Work out the finished part from the listing and answer in its coordinate system (mm). Face numbers are marked on the shaded views. A direction names the side the tool comes from. Round coordinates to 2 decimals unless told otherwise and drop trailing zeros. Loops run counter-clockwise (first coordinate to the right, second up) from the corner with the lowest first, then second, coordinate; pieces in that order, holes last. Notation, with made-up numbers: (-3, 33.25) - (10, 33.25) arc R16 cw to (10, 53.25) - close; hole circle Ø7 at (60, 45). An arc over 180 degrees is marked (long way). Answer as CSV lines item,"result". Start each with the question number.
Q1. For the marked faces 1 and 2, determine the directions among +Z, -Z, +X, -X, +Y, -Y from which every point of the face is accessible in a straight line to the end or side of a thin tool.
Q2. Section A-A on y = 0 is taken. Write down the section's boundary in (x, z).
Q3. Straight lines are drawn through the part: L1, parallel to Z at x = 14, y = 10.5; L2, parallel to Y at x = 0, z = 11; L3, parallel to Y at x = 0, z = 8. For each, find the intervals that lie inside material, in ascending order. Write a range as [from, to].
Q4. Each of these flat-tipped pins is pushed along its axis until it touches: pin 1 Ø3 at (x, z) = (1, 4) entering from -Y; pin 2 Ø4 at (y, z) = (-9.5, 8.5) entering from -X; pin 3 Ø1.5 at (x, y) = (-12, -11) entering from -Z. Where does it stop, or does it pass through?
Q5. Section C-C on z = 6 is taken. Write down the section's boundary in (x, y).
Q6. Section D-D on z = -8 is taken. Write down the section's boundary in (x, y), then the cut area to 3 significant figures.
Q7. Section B-B on x = 10 is taken. Write down the section's boundary in (y, z).
Q8. The mould has two halves that part along X. Classify the marked faces 3, 4 and 5: +X half, -X half, draft (parallel to the pull), parting line (faces both ways), or undercut.
```python
from build123d import *

# Parameters (mm, degrees)
SKETCH_1_R          = 18.5
SKETCH_1_R_2        = 3
EXTRUDE_1_DEPTH     = 14
SKETCH_2_R          = 18.5
SKETCH_2_R_2        = 17.3
CUT_EXTRUDE_1_DEPTH = 2.2
SKETCH_2_2_R        = 18.5
SKETCH_2_2_R_2      = 17.3
CUT_EXTRUDE_2_DEPTH = 0.8
SKETCH_2_4_R        = 18.5
SKETCH_2_4_R_2      = 17.3
CUT_EXTRUDE_3_DEPTH = 4
SKETCH_2_6_R        = 18.5
SKETCH_2_6_R_2      = 17.3
CUT_EXTRUDE_5_DEPTH = 3
SKETCH_3_R          = 7
EXTRUDE_3_DEPTH     = 5
SKETCH_4_R          = 6
EXTRUDE_4_DEPTH     = 12


with BuildPart() as part:
    # Sketch 1 → Extrude 1 (new body)
    with BuildSketch(Plane.XY):
        Circle(SKETCH_1_R)
        Circle(SKETCH_1_R_2, mode=Mode.SUBTRACT)
    extrude(amount=EXTRUDE_1_DEPTH)

    # Sketch 2 → Cut-Extrude 1 (cut)
    with BuildSketch(Plane.XY.offset(7.7)):
        Circle(SKETCH_2_R)
        Circle(SKETCH_2_R_2, mode=Mode.SUBTRACT)
    extrude(amount=-CUT_EXTRUDE_1_DEPTH, mode=Mode.SUBTRACT)

    # Sketch 2_2 → Cut-Extrude 2 (cut)
    with BuildSketch(Plane.XY.offset(7.7)):
        Circle(SKETCH_2_2_R)
        Circle(SKETCH_2_2_R_2, mode=Mode.SUBTRACT)
    extrude(amount=CUT_EXTRUDE_2_DEPTH, mode=Mode.SUBTRACT)

    # Sketch 2_4 → Cut-Extrude 3 (cut)
    with BuildSketch(Plane.XY.offset(7.7)):
        Circle(SKETCH_2_4_R)
        Circle(SKETCH_2_4_R_2, mode=Mode.SUBTRACT)
    extrude(amount=-CUT_EXTRUDE_3_DEPTH, mode=Mode.SUBTRACT)

    # Sketch 2_6 → Cut-Extrude 5 (cut)
    with BuildSketch(Plane.XY.offset(7.7)):
        Circle(SKETCH_2_6_R)
        Circle(SKETCH_2_6_R_2, mode=Mode.SUBTRACT)
    extrude(amount=CUT_EXTRUDE_5_DEPTH, mode=Mode.SUBTRACT)

    # Sketch 3 → Extrude 3 (add)
    with BuildSketch(Plane(origin=(0, 0, 0), x_dir=(-1, 0, 0), z_dir=(0, 0, -1))):
        Circle(SKETCH_3_R)
    extrude(amount=EXTRUDE_3_DEPTH)

    # Sketch 4 → Extrude 4 (add)
    with BuildSketch(Plane(origin=(0, 0, -5), x_dir=(-1, 0, 0), z_dir=(0, 0, -1))):
        Circle(SKETCH_4_R)
    extrude(amount=EXTRUDE_4_DEPTH)


solid = part.part
```
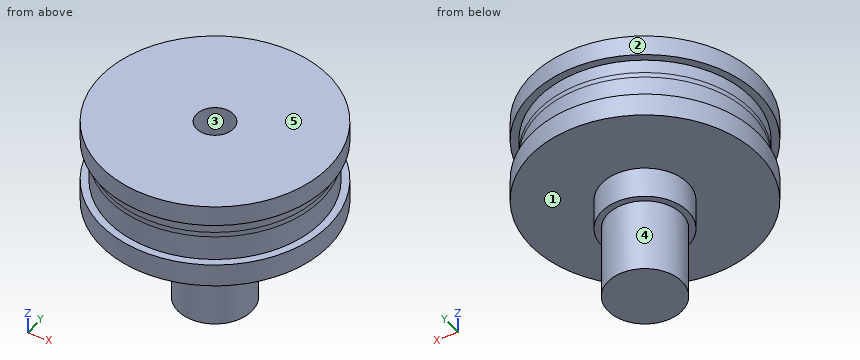
Findings:
1,face 1,"-Z"
1,face 2,"+Z, -Z"
2,outline,"(-18.5, 0) - (-7, 0) - (-7, -5) - (-6, -5) - (-6, -17) - (6, -17) - (6, -5) - (7, -5) - (7, 0) - (18.5, 0) - (18.5, 3.7) - (17.3, 3.7) - (17.3, 10.7) - (18.5, 10.7) - (18.5, 14) - (3, 14) - (3, 0) - (-3, 0) - (-3, 14) - (-18.5, 14) - (-18.5, 10.7) - (-17.3, 10.7) - (-17.3, 3.7) - (-18.5, 3.7) - close"
3,L1,"z = [0, 3.7], [10.7, 14]"
3,L2,"y = [-18.5, -3], [3, 18.5]"
3,L3,"y = [-17.3, -3], [3, 17.3]"
4,pin 1,"stops at y = -18.5"
4,pin 2,"stops at x = -15.59"
4,pin 3,"stops at z = 0"
5,outline,"circle Ø34.6 at (0, 0); hole circle Ø6 at (0, 0)"
6,outline,"circle Ø12 at (0, 0)"
6,area,"113 mm^2"
7,outline,"(-15.56, 0) - (15.56, 0) - (15.56, 3.7) - (14.12, 3.7) - (14.12, 10.7) - (15.56, 10.7) - (15.56, 14) - (-15.56, 14) - (-15.56, 10.7) - (-14.12, 10.7) - (-14.12, 3.7) - (-15.56, 3.7) - close"
8,face 3,"undercut"
8,face 4,"parting line"
8,face 5,"draft"
